Could you check a few things on this model? Use its own coordinates, in mm. Give positions to 0.01 mm unless a question says otherwise; leave off trailing zeros. Use one line per item in the form item = value.
```python
from build123d import *

# Parameters (mm, degrees)
SKETCH5_R           = 2.1
BOSS_EXTRUDE4_DEPTH = 780


with BuildPart() as part:
    # Sketch5 → Boss-Extrude4 (new body)
    with BuildSketch(Plane(origin=(0, 680, 0), x_dir=(1, 0, 0), z_dir=(0, 1, 0))):
        with BuildLine():
            Line((10.933291631, -2.510964723), (13.546664665, -2.510964723))
            Line((13.546664665, -2.510964723), (13.546664665, -4.150304529))
            Line((13.546664665, -4.150304529), (10.886004292, -6.810964917))
            Line((10.886004292, -6.810964917), (8.251433769, -6.810964917))
            Line((8.251433769, -6.810964917), (8.046664548, -7.015734138))
            Line((8.046664548, -7.015734138), (7.841895327, -6.810964917))
            Line((7.841895327, -6.810964917), (5.20732467, -6.810964917))
            Line((5.20732467, -6.810964917), (2.546664606, -4.150304933))
            Line((2.546664606, -4.150304933), (2.546664606, -2.510964723))
            Line((2.546664606, -2.510964723), (5.160037847, -2.510964723))
            Line((5.160037847, -2.510964723), (5.160037847, -2.404337587))
            Line((5.160037847, -2.404337587), (3.644466263, -0.888765902))
            ThreePointArc((3.644466263, -0.888765902), (3.447524808, -0.757173822), (3.215216519, -0.710964828))
            Line((3.215216519, -0.710964828), (-0.453335301, -0.710964828))
            ThreePointArc((-0.453335301, -0.710964828), (-1.51399556, -1.150304692), (-1.953335424, -2.210964951))
            Line((-1.953335424, -2.210964951), (-1.953335424, -5.810965145))
            ThreePointArc((-1.953335424, -5.810965145), (-1.920400619, -6.079855092), (-1.775534246, -6.308766076))
            Line((-1.775534246, -6.308766076), (-0.259962261, -7.82433806))
            Line((-0.259962261, -7.82433806), (-0.153335306, -7.82433806))
            Line((-0.153335306, -7.82433806), (-0.153335306, -5.210964844))
            Line((-0.153335306, -5.210964844), (1.48600445, -5.210964844))
            Line((1.48600445, -5.210964844), (4.146664635, -7.871625029))
            Line((4.146664635, -7.871625029), (4.146664635, -10.511096803))
            Line((4.146664635, -10.511096803), (4.346532653, -10.71096482))
            Line((4.346532653, -10.71096482), (4.146664635, -10.910832837))
            Line((4.146664635, -10.910832837), (4.146664635, -13.550304611))
            Line((4.146664635, -13.550304611), (1.486004498, -16.210964763))
            Line((1.486004498, -16.210964763), (-0.153335306, -16.210964763))
            Line((-0.153335306, -16.210964763), (-0.153335306, -13.597591958))
            Line((-0.153335306, -13.597591958), (-0.259962405, -13.597591958))
            Line((-0.259962405, -13.597591958), (-1.775534389, -15.113163943))
            ThreePointArc((-1.775534389, -15.113163943), (-1.907551313, -15.346664458), (-1.953335424, -15.610964996))
            Line((-1.953335424, -15.610964996), (-1.953335424, -19.210964568))
            ThreePointArc((-1.953335424, -19.210964568), (-1.513995592, -20.27162475), (-0.453335411, -20.710964582))
            Line((-0.453335411, -20.710964582), (3.215216577, -20.710964582))
            ThreePointArc((3.215216577, -20.710964582), (3.447524814, -20.6647556), (3.644466229, -20.533163554))
            Line((3.644466229, -20.533163554), (5.160037847, -19.017591936))
            Line((5.160037847, -19.017591936), (5.160037847, -18.910964955))
            Line((5.160037847, -18.910964955), (2.546664606, -18.910964955))
            Line((2.546664606, -18.910964955), (2.546664606, -17.271624993))
            Line((2.546664606, -17.271624993), (5.207324725, -14.610964873))
            Line((5.207324725, -14.610964873), (7.839690462, -14.610964873))
            Line((7.839690462, -14.610964873), (8.046664589, -14.406195535))
            Line((8.046664589, -14.406195535), (8.251433823, -14.610964873))
            Line((8.251433823, -14.610964873), (10.88600448, -14.610964873))
            Line((10.88600448, -14.610964873), (13.546664665, -17.271625059))
            Line((13.546664665, -17.271625059), (13.546664665, -18.910964955))
            Line((13.546664665, -18.910964955), (10.933291631, -18.910964955))
            Line((10.933291631, -18.910964955), (10.933291631, -19.017591953))
            Line((10.933291631, -19.017591953), (12.448863173, -20.533163494))
            ThreePointArc((12.448863173, -20.533163494), (12.645804654, -20.664755585), (12.878112969, -20.710964582))
            Line((12.878112969, -20.710964582), (16.546664468, -20.710964582))
            ThreePointArc((16.546664468, -20.710964582), (17.607324734, -20.271624715), (18.046664601, -19.210964449))
            Line((18.046664601, -19.210964449), (18.046664601, -15.542413801))
            ThreePointArc((18.046664601, -15.542413801), (18.000455626, -15.310105584), (17.868863597, -15.113164184))
            Line((17.868863597, -15.113164184), (16.353291472, -13.597591958))
            Line((16.353291472, -13.597591958), (16.246664762, -13.597591958))
            Line((16.246664762, -13.597591958), (16.246664762, -16.210964763))
            Line((16.246664762, -16.210964763), (14.607324803, -16.210964763))
            Line((14.607324803, -16.210964763), (11.94666457, -13.550304611))
            Line((11.94666457, -13.550304611), (11.94666457, -10.910832837))
            Line((11.94666457, -10.910832837), (11.746796552, -10.71096482))
            Line((11.746796552, -10.71096482), (11.94666457, -10.511096803))
            Line((11.94666457, -10.511096803), (11.94666457, -7.871625029))
            Line((11.94666457, -7.871625029), (14.607324755, -5.210964844))
            Line((14.607324755, -5.210964844), (16.246664762, -5.210964844))
            Line((16.246664762, -5.210964844), (16.246664762, -7.82433806))
            Line((16.246664762, -7.82433806), (16.353291723, -7.82433806))
            Line((16.353291723, -7.82433806), (17.868863593, -6.30876619))
            ThreePointArc((17.868863593, -6.30876619), (18.000455625, -6.111824797), (18.046664601, -5.879516585))
            Line((18.046664601, -5.879516585), (18.046664601, -2.210964977))
            ThreePointArc((18.046664601, -2.210964977), (17.60732473, -1.1503047), (16.546664453, -0.710964828))
            Line((16.546664453, -0.710964828), (12.87811338, -0.710964828))
            ThreePointArc((12.87811338, -0.710964828), (12.645805115, -0.757173815), (12.448863677, -0.888765877))
            Line((12.448863677, -0.888765877), (10.933291631, -2.404337922))
            Line((10.933291631, -2.404337922), (10.933291631, -2.510964723))
        make_face()
        with Locations(Location((8.046664646, -10.71096484, 0), (0, 0, 270))):
            Circle(SKETCH5_R, mode=Mode.SUBTRACT)
        Polygon((15.704247289, -4.138217153), (16.246664762, -4.138217153), (16.246664762, -2.510964723), (14.619412332, -2.510964723), (14.619412332, -3.053382543), align=None, mode=Mode.SUBTRACT)
        Polygon((16.246664762, -18.910964955), (16.246664762, -17.283712525), (15.704247289, -17.283712525), (14.619412332, -18.368547483), (14.619412332, -18.910964955), align=None, mode=Mode.SUBTRACT)
        Polygon((1.473917132, -3.053382195), (1.473917132, -2.510964723), (-0.153335306, -2.510964723), (-0.153335306, -4.138217153), (0.389082175, -4.138217153), align=None, mode=Mode.SUBTRACT)
        Polygon((1.473917132, -18.910964955), (1.473917132, -18.368547483), (0.389082175, -17.283712525), (-0.153335306, -17.283712525), (-0.153335306, -18.910964955), align=None, mode=Mode.SUBTRACT)
    extrude(amount=-BOSS_EXTRUDE4_DEPTH)


solid = part.part
```
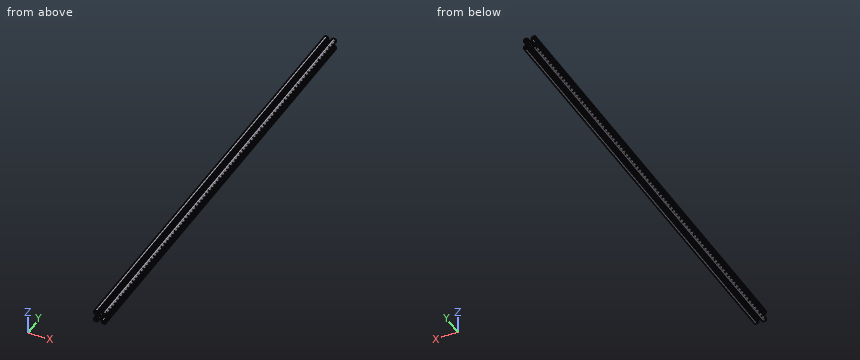
1. For pin 1 (3 mm diameter, centred on y = 439.5, z = 12.5, fed in from -X); pin 2 (2 mm diameter, centred on y = 457.5, z = 13, fed in from +X); pin 3 (1.3 mm diameter, centred on x = 9, y = 239, fed in from -Z); pin 4 (5 mm diameter, centred on x = 8.5, z = 17.5, fed in from +Y), each with a flat end and sliding along its axis, tell me the tip position at first contact or that it passes through.
Response values:
pin_1 = -0.66
pin_2 = 16.76
pin_3 = 6.81
pin_4 = through
2. If I drill on line 1 (Z direction, x = 0.5, y = 107.5); line 2 (Z direction, x = 0, y = 281.5); line 3 (X direction, y = 610, z = 3.5), over which ranges is the centre line in solid material (lowest first)? Write a range as from..to.
Response values:
line_1 = 0.71..2.51, 4.03..5.21, 16.21..17.39, 18.91..20.71
line_2 = 0.71..2.51, 4.14..5.21, 16.21..17.28, 18.91..20.71
line_3 = -1.95..-0.15, 1.03..2.55, 13.55..15.07, 16.25..18.05
3. Imagine slicing it at A-A, the plane y = 207.5. State how many separate pieces and enclosed holes the cut face has, and give its area (3 significant figures).
Response values:
separate_pieces = 1
enclosed_holes = 5
area = 162 mm²
